For this review, take the finished solid that the model builds, in its own axes (mm). A direction names the side the tool comes from. Give positions to 0.01 mm unless a question says otherwise; leave off trailing zeros. Loops run counter-clockwise (first coordinate to the right, second up) from the corner with the lowest first, then second, coordinate; pieces in that order, holes last. Notation, with made-up numbers: (18, 48.5) - (62, 48.5) arc R21 cw to (62, 86.5) - close; hole circle Ø9 at (-30.5, -11). An arc over 180 degrees is marked (long way). Answer in a Markdown table with one row per item.
```python
from build123d import *

# Parameters (mm, degrees)
F1_DEPTH = 1.5
F2_W     = 2.0366392564
F2_H     = 18.7370711938
F3_DEPTH = 3
F5_DEPTH = 1


# Not quite as in the source:
# - a feature names something its author has since deleted; it is built from what else it names


with BuildPart() as f1:
    # F0 (on Top) → F1 (new body)
    with BuildSketch(Plane.XY):
        Polygon((5.8843404986, 27.5437198579), (0, 55.8386333287), (-5.8843404986, 27.5437198579), (-5.8843404986, 0), (-48.9527061582, -25.7909391075), (-48.9527061582, -40.313988924), (-5.8843404986, -40.313988924), (-5.8843404986, -52.8338626027), (-30.9240873903, -63.3505582809), (-30.9240873903, -73.8672539592), (0, -73.8672539592), (30.9240873903, -73.8672539592), (30.9240873903, -63.3505582809), (5.8843404986, -52.8338626027), (5.8843404986, -40.313988924), (48.9527061582, -40.313988924), (48.9527061582, -25.7909391075), (5.8843404986, 0), align=None)
    extrude(amount=F1_DEPTH)

    # F2 (on face) → F3 (join)
    with BuildSketch(Plane.XY.offset(1.5)):
        with Locations((-1.0183196282, 20.6379326992)):
            Rectangle(F2_W, F2_H)
        with Locations((1.0183196282, 20.6379326992)):
            Rectangle(F2_W, F2_H)
    extrude(amount=F3_DEPTH)

    # F4 (on Right) → F5 (join)
    with BuildSketch(Plane.YZ):
        Polygon((-69.1700602547, 16.9719830155), (-73.7262964249, 0), (-48.7435348332, 0), (-62.592677772, 16.9719830155), align=None)
    extrude(amount=F5_DEPTH)


solid = f1.part
```
1. We need section C-C, the plane x = 8. Give the boundary of the cut face in (y, z).
Values:
| item | result |
|---|---|
| outline | (-73.87, 0) - (-53.72, 0) - (-53.72, 1.5) - (-73.87, 1.5) - close; (-40.31, 0) - (-1.27, 0) - (-1.27, 1.5) - (-40.31, 1.5) - close |
2. We need section A-A, the plane x = -18.5. Give the boundary of the cut face in (y, z).
Values:
| item | result |
|---|---|
| outline | (-73.87, 0) - (-58.13, 0) - (-58.13, 1.5) - (-73.87, 1.5) - close; (-40.31, 0) - (-7.55, 0) - (-7.55, 1.5) - (-40.31, 1.5) - close |
3. Mouldability with a two-part tool opening along Y and no side actions: class faces 6 (the face through (0.493, -56.192, 9.128)), 7 (the face through (0.49, -71.22, 9.34)), 8 (the face through (2.037, 21, 3)) as released by +Y, released by -Y, zero draft, split by the parting line, or undercut.
Values:
| item | result |
|---|---|
| face 6 | undercut |
| face 7 | released by -Y |
| face 8 | zero draft |
4. We need section D-D, the plane z = 10.5. Give the boundary of the cut face in (x, y).
Values:
| item | result |
|---|---|
| outline | (0, -70.91) - (1, -70.91) - (1, -57.31) - (0, -57.31) - close |
5. For faces 1 (the face through (1, -64, 8)), 2 (the face through (0, -64, 8)), 3 (the face through (0, 30.006, 3)), 4 (the face through (0, 11.269, 3)), 5 (the face through (-18.23, -58.02, 0.74)), list the 3-axis set-ups (+Z, -Z, +X, -X, +Y, -Y) from which the entire face can be reached by the end or side of a thin tool; tool diameter is ignored.
Values:
| item | result |
|---|---|
| face 1 | +Z, +X, -Y |
| face 2 | +Z, -X, -Y |
| face 3 | +Z, +X, -X, +Y |
| face 4 | +Z, +X, -X |
| face 5 | +Z, -Z, -X |
6. Wall thickness on line 1 (X direction, y = -63.5, z = 4.75); line 2 (Z direction, x = 9, y = -28); line 3 (Y direction, x = -32, z = 1): over which ranges is each line inside the solid? List them lowest first. Write a range as [from, to].
Values:
| item | result |
|---|---|
| line 1 | x = [0, 1] |
| line 2 | z = [0, 1.5] |
| line 3 | y = [-40.31, -15.64] |
7. Clearance check with flat-ended pins moving along their axes: pin 1 (0.8 mm diameter, centred on y = 17.5, z = 0.5, fed in from +X); pin 2 (6 mm diameter, centred on x = 6, y = -35, fed in from +Z); pin 3 (1.2 mm diameter, centred on y = -71, z = 1, fed in from +X); pin 4 (1.5 mm diameter, centred on x = 9, y = -39.5, fed in from -Z). State where each tip first meets the part, or that it passes through.
Values:
| item | result |
|---|---|
| pin 1 | stops at x = 5.88 |
| pin 2 | stops at z = 1.5 |
| pin 3 | stops at x = 30.92 |
| pin 4 | stops at z = 0 |
8. We need section B-B, the plane y = 14.5. Give the boundary of the cut face in (x, z).
Values:
| item | result |
|---|---|
| outline | (-5.88, 0) - (5.88, 0) - (5.88, 1.5) - (2.04, 1.5) - (2.04, 4.5) - (-2.04, 4.5) - (-2.04, 1.5) - (-5.88, 1.5) - close |
